Here's how the part is built. I have some questions about the finished solid (model axes, mm). Round coordinates to 2 decimals unless told otherwise and drop trailing zeros. Order: outer loops, then holes, each group sorted by start corner. A loop starts at its lowest first (then second) coordinate and runs counter-clockwise, first axis right, second up. Notation, with made-up numbers: (13, -24) -> (65, -24) arc R18 cw to (65, -11) -> close; hole circle Ø4 at (37.25, 87). An arc over 180 degrees is marked (long way). Answer in a Markdown table with one row per item.
```python
from build123d import *

# Parameters (mm, degrees)
F0_R     = 25
F1_DEPTH = 3.175


# Not quite as in the source:
# - a length typed as a fraction of an inch, garbled in the dataset ("3 / 203.2 mm" for 3/8 in), is restored


with BuildPart() as f1:
    # F0 (on Front) → F1 (new body)
    with BuildSketch(Plane.XZ):
        Polygon((-182.1372853069, 6.5356151886), (-178.9622853069, 6.5356151886), (125.8377146931, 6.5356151886), (129.0127146931, 6.5356151886), (129.0127146931, 31.9356151886), (125.8377146931, 31.9356151886), (125.8377146931, 57.3356151886), (129.0377632678, 57.3356151886), (129.0127146931, 82.7356151886), (125.8377146931, 82.7356151886), (125.8377146931, 108.1356151886), (129.0127146931, 108.1356151886), (129.0127146931, 111.3106151886), (125.8377146931, 111.3106151886), (100.4377146931, 111.3106151886), (100.4377146931, 108.1356151886), (75.0377146931, 108.1356151886), (75.0377146931, 111.3106151886), (49.6377146931, 111.3106151886), (49.6377146931, 108.1356151886), (24.2377146931, 108.1356151886), (24.2377146931, 111.3106151886), (-1.1622853069, 111.3106151886), (-1.1622853069, 108.1356151886), (-26.5622853069, 108.1356151886), (-26.5622853069, 111.3106151886), (-51.9622853069, 111.3106151886), (-51.9622853069, 108.1356151886), (-77.3622853069, 108.1356151886), (-77.3622853069, 111.3106151886), (-102.7622853069, 111.3106151886), (-102.7622853069, 108.1356151886), (-128.1622853069, 108.1356151886), (-128.1622853069, 111.3106151886), (-153.5622853069, 111.3106151886), (-153.5622853069, 108.1356151886), (-178.9622853069, 108.1356151886), (-178.9622853069, 82.7356151886), (-182.1372853069, 82.7356151886), (-182.1372853069, 57.3356151886), (-178.9622853069, 57.3356151886), (-178.9622853069, 31.9356151886), (-182.1372853069, 31.9356151886), align=None)
        with Locations((65.5590817332, 35.6867462397)):
            Circle(F0_R, mode=Mode.SUBTRACT)
    extrude(amount=F1_DEPTH)


solid = f1.part
```
1. Suppose I cut it at D-D on x = -158. Write out the boundary of the cut face in (y, z) (3 decimals).
Numbers:
| item | result |
|---|---|
| outline | (-3.175, 6.536) -> (0, 6.536) -> (0, 108.136) -> (-3.175, 108.136) -> close |
2. Suppose I cut it at C-C on z = 93. Write out the boundary of the cut face in (x, y) (3 decimals).
Numbers:
| item | result |
|---|---|
| outline | (-178.962, -3.175) -> (125.838, -3.175) -> (125.838, 0) -> (-178.962, 0) -> close |
3. For pin 1 Ø1 at (x, y) = (-181, -1.5) entering from +Z; pin 2 Ø1.6 at (x, y) = (-114.5, -2) entering from +Z; pin 3 Ø3 at (x, z) = (-36.5, 22) entering from +Y, each with a flat end and sliding along its axis, tell me the tip position at first contact or that it passes through.
Numbers:
| item | result |
|---|---|
| pin 1 | stops at z = 82.74 |
| pin 2 | stops at z = 108.14 |
| pin 3 | stops at y = 0 |
4. Please list where these lines run through material, in increasing order: line 1 along Z through (x, y) = (-74.5, -1.9); line 2 along X through (y, z) = (-0.4, 46.5); line 3 along X through (y, z) = (-0.85, 56).
Numbers:
| item | result |
|---|---|
| line 1 | z = 6.54 to 108.14 |
| line 2 | x = -178.96 to 43.02, 88.1 to 125.84 |
| line 3 | x = -178.96 to 50.99, 80.13 to 125.84 |
5. Suppose I cut it at B-B on z = 25. Write out the boundary of the cut face in (x, y) (3 decimals).
Numbers:
| item | result |
|---|---|
| outline | (-182.137, -3.175) -> (42.958, -3.175) -> (42.958, 0) -> (-182.137, 0) -> close; (88.16, -3.175) -> (129.013, -3.175) -> (129.013, 0) -> (88.16, 0) -> close |
6. Suppose I cut it at A-A on x = 58. Write out the boundary of the cut face in (y, z) (3 decimals), then the cut area to 3 significant figures.
Numbers:
| item | result |
|---|---|
| outline | (-3.175, 6.536) -> (0, 6.536) -> (0, 11.857) -> (-3.175, 11.857) -> close; (-3.175, 59.517) -> (0, 59.517) -> (0, 111.311) -> (-3.175, 111.311) -> close |
| area | 181 mm2 |
7. We'd pull the mould along X, two halves only. Please class faces 1 (the face through (60.14, -1.57, 11.28)), 2 (the face through (-29, -3.175, 60)): released by +X, released by -X, zero draft, split by the parting line, or undercut.
Numbers:
| item | result |
|---|---|
| face 1 | undercut |
| face 2 | zero draft |
